```python
from build123d import *

# Parameters (mm, degrees)
SKETCH_1_R         = 1.25
EXTRUDE_2_DEPTH    = 10
SKETCH1_W          = 5.221315892
SKETCH1_H          = 20.556
CUT_EXTRUDE1_DEPTH = 10
FILLET1_R          = 1
FILLET2_R          = 2.5


with BuildPart() as part:
    # Эскиз1 → Бобышка-Вытянуть2 (new body)
    with BuildSketch(Plane(origin=(0, 0, 0), x_dir=(1, 0, 0), z_dir=(0, 1, 0))):
        with BuildLine():
            Line((-6.75, -16.533718228), (-6.75, -17.533718228))
            Line((-6.75, -17.533718228), (1.25, -17.533718228))
            Line((1.25, -17.533718228), (5.75, -17.533718228))
            ThreePointArc((5.75, -17.533718228), (6.457106781, -17.240825009), (6.75, -16.533718228))
            Line((6.75, -16.533718228), (6.75, 16.538507887))
            ThreePointArc((6.75, 16.538507887), (6.457106781, 17.245614668), (5.75, 17.538507887))
            Line((5.75, 17.538507887), (-5.75, 17.538507887))
            ThreePointArc((-5.75, 17.538507887), (-6.457106781, 17.245614668), (-6.75, 16.538507887))
            Line((-6.75, 16.538507887), (-6.75, 5.538507887))
            ThreePointArc((-6.75, 5.538507887), (-6.457106781, 4.831401106), (-5.75, 4.538507887))
            Line((-5.75, 4.538507887), (-5.746697715, 4.538507887))
            ThreePointArc((-5.746697715, 4.538507887), (-5.039590934, 4.245614668), (-4.746697715, 3.538507887))
            Line((-4.746697715, 3.538507887), (-4.746697715, -8.461492113))
            ThreePointArc((-4.746697715, -8.461492113), (-5.039590934, -9.168598894), (-5.746697715, -9.461492113))
            Line((-5.746697715, -9.461492113), (-5.75, -9.461492113))
            ThreePointArc((-5.75, -9.461492113), (-6.457106781, -9.754385332), (-6.75, -10.461492113))
            Line((-6.75, -10.461492113), (-6.75, -16.533718228))
        make_face()
        with Locations(Location((-2.75, 13.538507887, 0), (0, 0, 270))):
            Circle(SKETCH_1_R, mode=Mode.SUBTRACT)
        with Locations(Location((4.25, -13.316820051, 0), (0, 0, 270))):
            Circle(SKETCH_1_R, mode=Mode.SUBTRACT)
    extrude(amount=EXTRUDE_2_DEPTH)

    # Sketch1 → Cut-Extrude1 (cut)
    with BuildSketch(Plane.XZ):
        with Locations((-5.139342054, 2.709492113)):
            Rectangle(SKETCH1_W, SKETCH1_H)
    extrude(amount=-CUT_EXTRUDE1_DEPTH, mode=Mode.SUBTRACT)

    # Fillet1
    fillet1_edges = [part.edges().sort_by_distance(p)[0] for p in [
        (-6.75, 5, 17.533718228),
    ]]
    fillet(fillet1_edges, radius=FILLET1_R)

    # Fillet2
    fillet2_edges = [part.edges().sort_by_distance(p)[0] for p in [
        (-2.528684108, 5, -7.568507887),
        (-2.528684108, 5, 12.987492113),
    ]]
    fillet(fillet2_edges, radius=FILLET2_R)


solid = part.part
```
Design review of the part built by this model. Coordinates are the model's own, in mm. A direction names the side the tool comes from. Give positions to 0.01 mm unless a question says otherwise; leave off trailing zeros. Order: outer loops, then holes, each group sorted by start corner. A loop starts at its lowest first (then second) coordinate and runs counter-clockwise, first axis right, second up. Notation, with made-up numbers: (68.5, 45) - (115.5, 45) arc R22 cw to (115.5, 60) - close; hole circle Ø5 at (63, 23.5). An arc over 180 degrees is marked (long way). Use a Markdown table: item, result. Add a question column.
(1) Add section C-C on z = -2. Give the boundary of the cut face in (x, y).
(2) Wall thickness on probe 1 along X at (y, z) = (6.25, 2); probe 2 along Z at (x, y) = (-5, 5.5); probe 3 along Z at (x, y) = (-2, 6.75): over which ranges is each line inside the solid? List them lowest first. Write a range as [from, to].
(3) Add section A-A on x = 4.25. Give the boundary of the cut face in (y, z).
(4) Add section B-B on y = 4.75. Give the boundary of the cut face in (x, z).
(5) Machinability: for faces 1 (the face through (-6.4, 4.9, -17.3)), 2 (the face through (-6, 5, -7.569)), which of the approach directions +Z, -Z, +X, -X, +Y, -Y give a long, thin tool a straight path to every point of the face, cutting with its end or side? Answer none if there is none.
(6) Clearance check with a flat-ended pin moving along its axis: P1, Ø2, axis at x = -2.75, z = -13.54, coming from the -Y side. State where the tip first meets the part, or that it passes through.
(7) Mouldability with a two-part tool opening along X and no side actions: class faces 3 (the face through (-6.45, 5.07, 17.25)), 4 (the face through (-2.375, 4.93, -12.346)), 5 (the face through (0, 5, -17.539)) as +X half, -X half, draft (parallel to the pull), parting line (faces both ways), or undercut.
(8) Add section D-D on z = -6.5. Give the boundary of the cut face in (x, y), then the cut area to 3 significant figures.
Report:
| question | item | result |
|---|---|---|
| 1 | outline | (-2.53, 0) - (6.75, 0) - (6.75, 10) - (-2.53, 10) - close |
| 2 | probe 1 | x = [-2.53, 6.75] |
| 2 | probe 2 | z = [-17.54, -7.57], [12.99, 17.53] |
| 2 | probe 3 | z = [-17.54, -14.54], [-12.54, 17.53] |
| 3 | outline | (0, -17.54) - (10, -17.54) - (10, 12.07) - (0, 12.07) - close; (0, 14.57) - (10, 14.57) - (10, 17.53) - (0, 17.53) - close |
| 4 | outline | (-6.75, -16.54) arc R1 ccw to (-5.75, -17.54) - (5.75, -17.54) arc R1 ccw to (6.75, -16.54) - (6.75, 16.53) arc R1 ccw to (5.75, 17.53) - (-5.75, 17.53) arc R1 ccw to (-6.75, 16.53) - (-6.75, 12.99) - (-5.03, 12.99) arc R2.5 cw to (-2.53, 10.49) - (-2.53, -5.07) arc R2.5 cw to (-5.03, -7.57) - (-6.75, -7.57) - close; hole circle Ø2.5 at (-2.75, -13.54); hole circle Ø2.5 at (4.25, 13.32) |
| 5 | face 1 | -Z, -X, +Y, -Y |
| 5 | face 2 | -X, +Y, -Y |
| 6 | P1 | passes through |
| 7 | face 3 | -X half |
| 7 | face 4 | undercut |
| 7 | face 5 | draft |
| 8 | outline | (-2.98, 0) - (6.75, 0) - (6.75, 10) - (-2.98, 10) - close |
| 8 | area | 97.3 mm² |
